Geometry: see drawing. Coordinates: mm, zero at the bounding-box minimum. A direction names the side the tool comes from. Coordinates: 2 decimals unless noted, no trailing zeros. Loops run counter-clockwise (first coordinate to the right, second up) from the corner with the lowest first, then second, coordinate; pieces in that order, holes last. Notation, with made-up numbers: (65, 62) - (71, 62) arc R13 ccw to (71, 74) - close; hole circle Ø6 at (7.5, 23). An arc over 180 degrees is marked (long way). Use a Markdown table: item, result. Add a question column.
1. Section query A-A on z = 2.4. Return the cut outline in (x, y).
2. Section query D-D on y = 1.75. Return the cut outline in (x, z), then the cut area to 3 significant figures.
3. Contact query for flat-ended pins moving along their axis: P1, Ø1, axis at y = 1, z = 1.5, coming from the +X side; P2, Ø1.6, axis at y = 0.5, z = 1.5, coming from the -X side; P3, Ø0.6, axis at x = 2.5, y = 1, coming from the +Z side. Output: stop coordinate, or through.
4. Section query C-C on y = 10.5. Return the cut outline in (x, z), then the cut area to 3 significant figures.
5. Section query B-B on x = 2. Return the cut outline in (y, z).
6. Access query for the marked faces 1, 2, 3 and 4. Directions: +Z, -Z, +X, -X, +Y, -Y. A direction counts if a zero-diameter tool reaches every point of the face in a straight line with its end or side. Return the directions, or none.
7. Ray query, L1, parallel to Z at x = 2.1, y = 2.5; L2, parallel to Y at x = 3.55, z = 1.15; L3, parallel to Z at x = 0.9, y = 1.25. Return the intervals inside material, ascending. Write a range as [from, to].
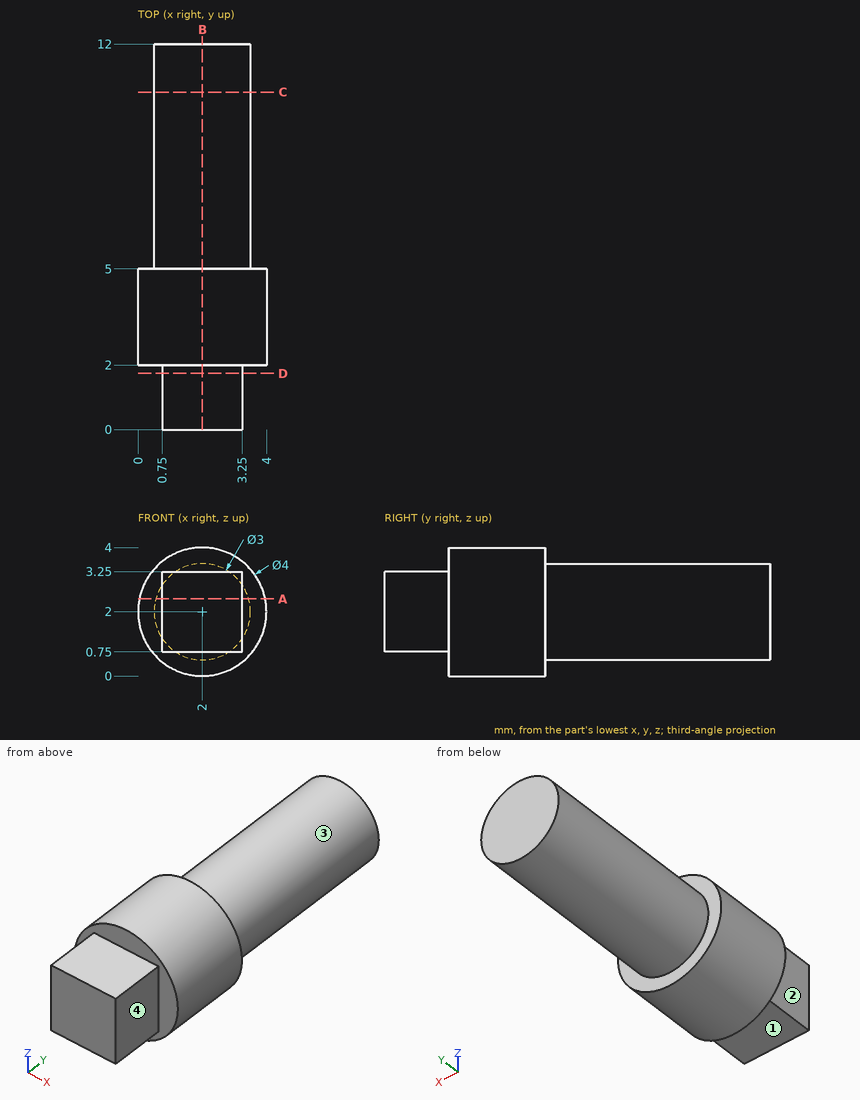
Resolved:
| question | item | result |
|---|---|---|
| 1 | outline | (0.04, 2) - (0.75, 2) - (0.75, 0) - (3.25, 0) - (3.25, 2) - (3.96, 2) - (3.96, 5) - (3.45, 5) - (3.45, 12) - (0.55, 12) - (0.55, 5) - (0.04, 5) - close |
| 2 | outline | (0.75, 0.75) - (3.25, 0.75) - (3.25, 3.25) - (0.75, 3.25) - close |
| 2 | area | 6.25 mm² |
| 3 | P1 | x = 3.25 |
| 3 | P2 | x = 0.75 |
| 3 | P3 | z = 3.25 |
| 4 | outline | circle Ø3 at (2, 2) |
| 4 | area | 7.07 mm² |
| 5 | outline | (0, 0.75) - (2, 0.75) - (2, 0) - (5, 0) - (5, 0.5) - (12, 0.5) - (12, 3.5) - (5, 3.5) - (5, 4) - (2, 4) - (2, 3.25) - (0, 3.25) - close |
| 6 | face 1 | -Z, +X, -X, -Y |
| 6 | face 2 | +Z, -Z, -X, -Y |
| 6 | face 3 | +Y |
| 6 | face 4 | +Z, -Z, +X, -Y |
| 7 | L1 | [0, 4] |
| 7 | L2 | [2, 5] |
| 7 | L3 | [0.75, 3.25] |
